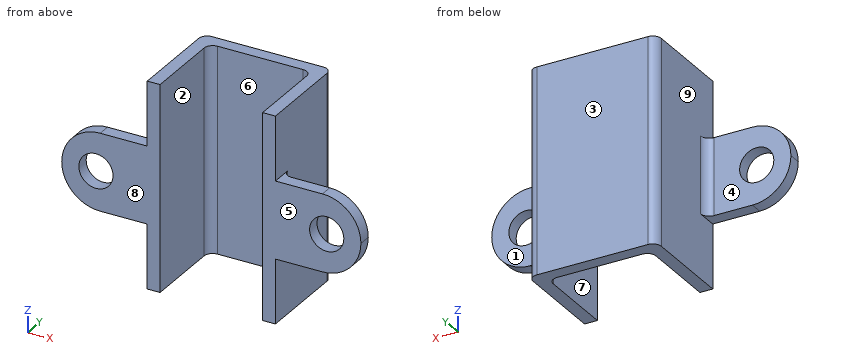
from build123d import *

# Parameters (mm, degrees)
SALIENTE_EXTRUIR2_DEPTH = 12
CROQUIS4_W              = 10
CROQUIS4_H              = 7.5
CORTAR_EXTRUIR2_DEPTH   = 24.457408211
CROQUIS6_R              = 2
CORTAR_EXTRUIR3_DEPTH   = 24.457408211
CORTAR_EXTRUIR4_DEPTH   = 24.457408211
REDONDEO1_R             = 1
REDONDEO2_R             = 1
REDONDEO3_R             = 1
REDONDEO4_R             = 1
REDONDEO5_R             = 1
REDONDEO6_R             = 1


with BuildPart() as part:
    # Croquis1 → Saliente-Extruir2 (new, symmetric)
    with BuildSketch(Plane.XY):
        Polygon((-17.5, -11.5), (-17.5, -10), (-7.5, -10), (-7.5, 0), (7.5, 0), (7.5, -10), (17.5, -10), (17.5, -11.5), (6, -11.5), (6, -1.5), (-6, -1.5), (-6, -11.5), align=None)
    extrude(amount=SALIENTE_EXTRUIR2_DEPTH, both=True)

    # Croquis4 → Cortar-Extruir2 (cut, through all)
    with BuildSketch(Plane(origin=(0, -10, 0), x_dir=(1, 0, 0), z_dir=(0, 1, 0))):
        with Locations((-12.5, 8.25)):
            Rectangle(CROQUIS4_W, CROQUIS4_H)
        with Locations((12.5, 8.25)):
            Rectangle(CROQUIS4_W, CROQUIS4_H)
        with Locations((12.5, -8.25)):
            Rectangle(CROQUIS4_W, CROQUIS4_H)
        with Locations((-12.5, -8.25)):
            Rectangle(CROQUIS4_W, CROQUIS4_H)
    extrude(amount=-CORTAR_EXTRUIR2_DEPTH, mode=Mode.SUBTRACT)

    # Croquis6 → Cortar-Extruir3 (cut, through all)
    with BuildSketch(Plane(origin=(0, -10, 0), x_dir=(1, 0, 0), z_dir=(0, 1, 0))):
        with Locations(Location((-13.5, 0, 0), (0, 0, 270))):
            Circle(CROQUIS6_R)
        with Locations(Location((13.5, 0, 0), (0, 0, 270))):
            Circle(CROQUIS6_R)
    extrude(amount=-CORTAR_EXTRUIR3_DEPTH, mode=Mode.SUBTRACT)

    # Croquis7 → Cortar-Extruir4 (cut, through all)
    with BuildSketch(Plane(origin=(0, -10, 0), x_dir=(1, 0, 0), z_dir=(0, 1, 0))):
        with BuildLine():
            ThreePointArc((-17.5, 0), (-16.181980515, 3.181980515), (-13, 4.5))
            Line((-13, 4.5), (-17.5, 4.5))
            Line((-17.5, 4.5), (-17.5, 0))
        make_face()
        with BuildLine():
            ThreePointArc((-13, -4.5), (-16.181980515, -3.181980515), (-17.5, 0))
            Line((-17.5, 0), (-17.5, -4.5))
            Line((-17.5, -4.5), (-13, -4.5))
        make_face()
        with BuildLine():
            Line((17.5, 4.5), (13, 4.5))
            ThreePointArc((13, 4.5), (16.181980515, 3.181980515), (17.5, 0))
            Line((17.5, 0), (17.5, 4.5))
        make_face()
        with BuildLine():
            Line((17.5, -4.5), (17.5, 0))
            ThreePointArc((17.5, 0), (16.181980515, -3.181980515), (13, -4.5))
            Line((13, -4.5), (17.5, -4.5))
        make_face()
    extrude(amount=-CORTAR_EXTRUIR4_DEPTH, mode=Mode.SUBTRACT)

    # Redondeo1
    redondeo1_edges = [part.edges().sort_by_distance(p)[0] for p in [
        (-7.5, -10, 0),
    ]]
    fillet(redondeo1_edges, radius=REDONDEO1_R)

    # Redondeo2
    redondeo2_edges = [part.edges().sort_by_distance(p)[0] for p in [
        (7.5, -10, 0),
    ]]
    fillet(redondeo2_edges, radius=REDONDEO2_R)

    # Redondeo3
    redondeo3_edges = [part.edges().sort_by_distance(p)[0] for p in [
        (-6, -1.5, 0),
    ]]
    fillet(redondeo3_edges, radius=REDONDEO3_R)

    # Redondeo4
    redondeo4_edges = [part.edges().sort_by_distance(p)[0] for p in [
        (6, -1.5, 0),
    ]]
    fillet(redondeo4_edges, radius=REDONDEO4_R)

    # Redondeo5
    redondeo5_edges = [part.edges().sort_by_distance(p)[0] for p in [
        (-7.5, 0, 0),
    ]]
    fillet(redondeo5_edges, radius=REDONDEO5_R)

    # Redondeo6
    redondeo6_edges = [part.edges().sort_by_distance(p)[0] for p in [
        (7.5, 0, 0),
    ]]
    fillet(redondeo6_edges, radius=REDONDEO6_R)


solid = part.part
Here's how the part is built. I have some questions about the finished solid (model axes, mm). Face numbers are marked on the shaded views. A direction names the side the tool comes from. Round coordinates to 2 decimals unless told otherwise and drop trailing zeros. Order: outer loops, then holes, each group sorted by start corner. A loop starts at its lowest first (then second) coordinate and runs counter-clockwise, first axis right, second up. Notation, with made-up numbers: (54, -22.5) -> (80, -22.5) arc R37 ccw to (80, 16.5) -> close; hole circle Ø7 at (53, -10.5). An arc over 180 degrees is marked (long way). Use CSV: the item, a comma, the result in double quotes.
1. Which directions (+Z, -Z, +X, -X, +Y, -Y) give clear straight access to the entire face, cutting with the end or side of a thin tool? Please do the marked faces 1, 2, 3, 4 and 5.
Recorded:
face 1,"+Z, -Z, +X, +Y"
face 2,"+Z, -Z, -Y"
face 3,"+Z, -Z, +X, -X, +Y"
face 4,"+Z, -Z, -X, +Y"
face 5,"+Z, -Z, +X, -X, -Y"
2. I want a section at D-D on y = -9.5. List the corners of the cut face in (x, z) for me.
Recorded:
outline,"(-7.63, -4.5) -> (-7.5, -4.5) -> (-7.5, -12) -> (-6, -12) -> (-6, 12) -> (-7.5, 12) -> (-7.5, 4.5) -> (-7.63, 4.5) -> close; (6, -12) -> (7.5, -12) -> (7.5, -4.5) -> (7.63, -4.5) -> (7.63, 4.5) -> (7.5, 4.5) -> (7.5, 12) -> (6, 12) -> close"
3. Thinking about a two-plate mould opening in X: for the marked faces 6, 7, 8 and 9, which applies, pulls with the +X half, pulls with the -X half, needs draft (parallel to the pull), parting line crosses it, or undercut?
Recorded:
face 6,"undercut"
face 7,"undercut"
face 8,"needs draft"
face 9,"pulls with the -X half"
4. I want a section at A-A on y = -5.75. List the corners of the cut face in (x, z) for me, and give its area (3 significant figures).
Recorded:
outline,"(-7.5, -12) -> (-6, -12) -> (-6, 12) -> (-7.5, 12) -> close; (6, -12) -> (7.5, -12) -> (7.5, 12) -> (6, 12) -> close"
area,"72.0 mm2"
5. I need wall thicknesses on line 1 along X through (y, z) = (-5.25, -6.75); line 2 along Y through (x, z) = (0, 10.5); line 3 along Y through (x, z) = (11, -2.5). Which ranges of each line are inside material? Lowest first, please.
Recorded:
line 1,"x = -7.5 to -6, 6 to 7.5"
line 2,"y = -1.5 to 0"
line 3,"y = -11.5 to -10"
6. I want a section at C-C on z = -6.5. List the corners of the cut face in (x, y) for me, and give its area (3 significant figures).
Recorded:
outline,"(-7.5, -11.5) -> (-6, -11.5) -> (-6, -2.5) arc R1 cw to (-5, -1.5) -> (5, -1.5) arc R1 cw to (6, -2.5) -> (6, -11.5) -> (7.5, -11.5) -> (7.5, -1) arc R1 ccw to (6.5, 0) -> (-6.5, 0) arc R1 ccw to (-7.5, -1) -> close"
area,"52.5 mm2"
7. I want a section at B-B on x = 13.5. List the corners of the cut face in (y, z) for me, and give its area (3 significant figures).
Recorded:
outline,"(-11.5, -4.47) -> (-10, -4.47) -> (-10, -2) -> (-11.5, -2) -> close; (-11.5, 2) -> (-10, 2) -> (-10, 4.47) -> (-11.5, 4.47) -> close"
area,"7.42 mm2"
8. I'm going to push flat-ended pins straight in: P1, Ø5, axis at y = -4.5, z = 4.5, coming from the +X side; P2, Ø1, axis at y = -9, z = 4.5, coming from the +X side; P3, Ø2, axis at x = -10.5, y = -10.5, coming from the +Z side. Where does each tip first touch, or does it pass through?
Recorded:
P1,"stops at x = 7.5"
P2,"stops at x = 7.63"
P3,"stops at z = 4.5"
